Work out the finished part from the listing and answer in its coordinate system (mm). Round coordinates to 2 decimals unless told otherwise and drop trailing zeros. Put each result on its own line as item: value.
```python
from build123d import *

# Parameters (mm, degrees)
SKETCH3_R          = 85.725
SKETCH3_R_2        = 1.5875
BASE_EXTRUDE_DEPTH = 15.875
FILLET2_R          = 6.35
FILLET3_R          = 3.175
FILLET4_R          = 2.032


with BuildPart() as part:
    # Sketch3 → Base-Extrude (new body)
    with BuildSketch(Plane(origin=(0, 0, 0), x_dir=(1, 0, 0), z_dir=(0, 1, 0))):
        with Locations(Location((0, 0, 0), (0, 0, 270))):
            Circle(SKETCH3_R)
        with Locations(Location((0, 0, 0), (0, 0, 270))):
            Circle(SKETCH3_R_2, mode=Mode.SUBTRACT)
        with Locations(Location((0, 76.2, 0), (0, 0, 270))):
            Circle(SKETCH3_R_2, mode=Mode.SUBTRACT)
    extrude(amount=BASE_EXTRUDE_DEPTH)

    # Fillet2
    fillet2_edges = [part.edges().sort_by_distance(p)[0] for p in [
        (0, 15.875, -85.725),
    ]]
    fillet(fillet2_edges, radius=FILLET2_R)

    # Fillet3
    fillet3_edges = [part.edges().sort_by_distance(p)[0] for p in [
        (0, 15.875, -1.5875),
    ]]
    fillet(fillet3_edges, radius=FILLET3_R)

    # Fillet4
    fillet4_edges = [part.edges().sort_by_distance(p)[0] for p in [
        (0, 15.875, -77.7875),
    ]]
    fillet(fillet4_edges, radius=FILLET4_R)


solid = part.part
```
1) A cutting plane is placed at A-A on y = 4.75. Give the number of separate pieces and of enclosed holes in the cut face, then the cut area to 3 significant figures.
Findings below:
separate pieces: 1
enclosed holes: 2
area: 23,100 mm2
2) Straight lines are drawn through the part: L1, parallel to Z at x = 1, y = 13; L2, parallel to X at y = 7, z = 0 (1 decimal); L3, parallel to X at y = 5.25, z = -76.2. For each, find the intervals that lie inside material, in ascending order. Write a range as from..to.
Findings below:
L1: z = -84.68..-77.43, -74.97..-1.25, 1.25..84.68
L2: x = -85.7..-1.6, 1.6..85.7
L3: x = -39.27..-1.59, 1.59..39.27
3) Given pin 1 Ø1.5 at (x, y) = (-55, 13.5) entering from +Z; pin 2 Ø1.5 at (y, z) = (1.5, 20.5) entering from -X; pin 3 Ø4 at (y, z) = (4.5, -31.5) entering from +X, each flat-ended and moving along its own axis, determine where each tip first touches the part or whether it passes through.
Findings below:
pin 1: stops at z = 64.87
pin 2: stops at x = -83.42
pin 3: stops at x = 80.49
